Here's how the part is built. I have some questions about the finished solid (model axes, mm). Give positions to 0.01 mm unless a question says otherwise; leave off trailing zeros. Loops run counter-clockwise (first coordinate to the right, second up) from the corner with the lowest first, then second, coordinate; pieces in that order, holes last. Notation, with made-up numbers: (-11, -26.75) -> (34, -26.75) arc R30 ccw to (34, 1.25) -> close; hole circle Ø2 at (11, 23.5). An arc over 180 degrees is marked (long way). Answer in a Markdown table with one row per item. Add a question column.
Item 1: If we section it at A-A (y = 4): Write out the boundary of the cut face in (x, z), then the cut area to 4 significant figures.
Item 2: If we section it at B-B (z = 1.15): Write out the boundary of the cut face in (x, y).
Item 3: If we section it at C-C (x = -14): Write out the boundary of the cut face in (y, z).
Item 4: If I drill on line 1 (Y direction, x = -29, z = 1.6); line 2 (Y direction, x = 4.5, z = 0.5); line 3 (X direction, y = 3, z = 0.3), over which ranges is the centre line in solid material (lowest first)?
Item 5: If we section it at D-D (y = -0.15): Write out the boundary of the cut face in (x, z), then the cut area to 4 significant figures.
Item 6: For P1, Ø2.5, axis at x = -29, y = -0.15, coming from the -Z side, with a flat end and sliding along its axis, tell me the tip position at first contact or that it passes through.
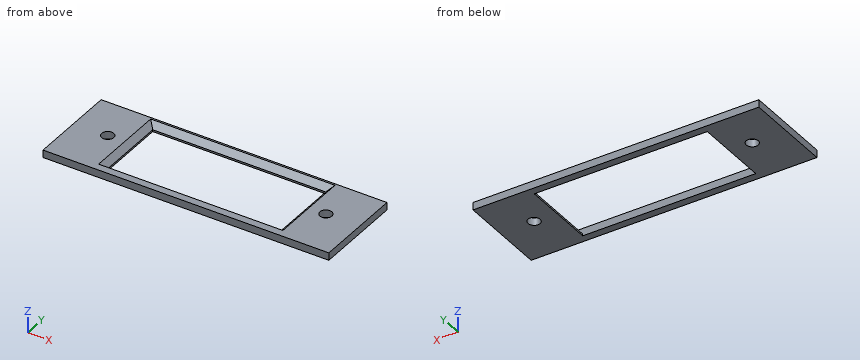
Autodesk Inventor part; units mm, degrees
ref_plane "YZ Plane" through (0, 0, 0) normal (1, 0, 0) x (0, 1, 0)
ref_plane "XZ Plane" through (0, 0, 0) normal (0, 1, 0) x (-1, 0, 0)
ref_plane "XY Plane" through (0, 0, 0) normal (0, 0, 1) x (1, 0, 0)
ref_plane "Arbeitsebene1" through (0, 0, 0) normal (0, 0, 1) x (1, 0, 0)
sketch "Skizze1" plane through (0, 0, 0) normal (0, 0, 1) x (1, 0, 0)
  circle A0 centre (12, 2.9) radius 1.5
  circle A1 centre (-12, 2.9) radius 1.5
  line L0 (38, 12.9) -> (-38, 12.9)
  line L1 (38, -12.9) -> (38, 12.9)
  line L2 (-38, -12.9) -> (38, -12.9)
  line L3 (-38, 12.9) -> (-38, -12.9)
  line L4 (-38, -12.9) -> (38, -12.9)
  line L5 (38, -12.9) -> (38, 11.1)
  line L6 (38, 11.1) -> (-38, 11.1)
  line L7 (-38, 11.1) -> (-38, -12.9)
  line L8 (-36, 9.1) -> (36, 9.1)
  line L9 (36, 9.1) -> (36, -10.9)
  line L10 (36, -10.9) -> (-36, -10.9)
  line L11 (-36, -10.9) -> (-36, 9.1)
  line L12 (-36, 9.1) -> (-23, 9.1)
  line L13 (-23, 9.1) -> (-23, -10.9)
  line L14 (-23, -10.9) -> (-36, -10.9)
  line L15 (-36, -10.9) -> (-36, 9.1)
  line L16 (36, 9.1) -> (23, 9.1)
  line L17 (23, 9.1) -> (23, -10.9)
  line L18 (23, -10.9) -> (36, -10.9)
  line L19 (36, -10.9) -> (36, 9.1)
  point P0 (-23, 9.1)
  point P1 (23, 9.1)
  dimension "d6" = 24
  dimension "d7" = 2
  dimension "d8" = 13
  dimension "d9" = 13
extrude "Extrusion1" add sketch "Skizze1" along normal blind 2 contours L1 L2 L3 L6 | L8 L13 L10 L11 | L8 L9 L10 L17
chamfer "Fasen1" distance 1.5 angle 45 3 edges at (0, 9.1, 2) (23, -0.9, 2) (-23, -0.9, 2)
sketch "Skizze2" plane through (0, 0, 2) normal (0, 0, 1) x (1, 0, 0)
  line L0 (24.5, -10.9) -> (-24.5, -10.9)
  line L1 (-24.5, 10.6) -> (-24.5, -10.9)
  line L2 (24.5, 10.6) -> (-24.5, 10.6)
  line L3 (24.5, -10.9) -> (24.5, 10.6)
  line L4 (-38, 11.1) -> (-38, -12.9)
  line L5 (-38, -12.9) -> (38, -12.9)
  line L6 (38, -12.9) -> (38, 11.1)
  line L7 (38, 11.1) -> (-38, 11.1)
  circle A0 centre (-12, 2.9) radius 1.5
  circle A1 centre (-29, -0.15) radius 1.6
  circle A2 centre (29, -0.15) radius 1.6
  point P0 (0, 0)
  dimension "d10" = 3.2
  dimension "d11" = 3.2
  dimension "d12" = 9
  dimension "d13" = 9
extrude "Extrusion2" cut sketch "Skizze2" against normal blind 10 contours A1 | A2
properties part number "00_coverglass_frame"
Recorded:
| question | item | result |
|---|---|---|
| 1 | outline | (-38, 0) -> (-23, 0) -> (-23, 0.5) -> (-24.5, 2) -> (-38, 2) -> close; (23, 0) -> (38, 0) -> (38, 2) -> (24.5, 2) -> (23, 0.5) -> close |
| 1 | area | 57.75 mm^2 |
| 2 | outline | (-38, -12.9) -> (38, -12.9) -> (38, 11.1) -> (-38, 11.1) -> close; hole circle Ø3.2 at (-29, -0.15); hole (-23.65, -10.9) -> (23.65, -10.9) -> (23.65, 9.75) -> (-23.65, 9.75) -> close; hole circle Ø3.2 at (29, -0.15) |
| 3 | outline | (-12.9, 0) -> (-10.9, 0) -> (-10.9, 2) -> (-12.9, 2) -> close; (9.1, 0) -> (11.1, 0) -> (11.1, 2) -> (10.6, 2) -> (9.1, 0.5) -> close |
| 4 | line 1 | y = -12.9 to -1.75, 1.45 to 11.1 |
| 4 | line 2 | y = -12.9 to -10.9, 9.1 to 11.1 |
| 4 | line 3 | x = -38 to -23, 23 to 38 |
| 5 | outline | (-38, 0) -> (-30.6, 0) -> (-30.6, 2) -> (-38, 2) -> close; (-27.4, 0) -> (-23, 0) -> (-23, 0.5) -> (-24.5, 2) -> (-27.4, 2) -> close; (23, 0) -> (27.4, 0) -> (27.4, 2) -> (24.5, 2) -> (23, 0.5) -> close; (30.6, 0) -> (38, 0) -> (38, 2) -> (30.6, 2) -> close |
| 5 | area | 44.95 mm^2 |
| 6 | P1 | passes through |
